Verification items for the finished model (mm, model axes). A direction names the side the tool comes from. Give positions to 0.01 mm unless a question says otherwise; leave off trailing zeros. Loops run counter-clockwise (first coordinate to the right, second up) from the corner with the lowest first, then second, coordinate; pieces in that order, holes last. Notation, with made-up numbers: (-19, 79) - (-4, 79) arc R5 cw to (-4, 86) - close; hole circle Ø1 at (21.5, 74.25). An arc over 180 degrees is marked (long way). Use one line per item in the form item = value.
```python
from build123d import *

# Parameters (mm, degrees)
HOLE_WIZARD_M6_1_D     = 5
HOLE_WIZARD_M6_1_DEPTH = 15
HOLE_WIZARD_M6_1_TIP   = 1.502151548
CHAMFER_1_SIZE         = 0.2


with BuildPart() as part:
    # 草图1 → 旋转1 (revolve)
    with BuildSketch(Plane.XY):
        Polygon((0, 0), (7.5, 0), (7.5, 70.5), (4.5, 70.5), (4.5, 72.5), (5, 72.5), (5, 76.267949192), (4, 80), (0, 80), align=None)
    revolve(axis=Axis((0, -1000, 0), (0, 1, 0)))

    # M6 螺纹孔1
    with Locations(Plane(origin=(0, 0, 0), x_dir=(-1, 0, 0), z_dir=(0, -1, 0))):
        with Locations((0, 0)):
            Hole(HOLE_WIZARD_M6_1_D / 2, depth=HOLE_WIZARD_M6_1_DEPTH)
            with Locations((0, 0, -(HOLE_WIZARD_M6_1_DEPTH + HOLE_WIZARD_M6_1_TIP / 2))):  # 118° drill point
                Cone(0, HOLE_WIZARD_M6_1_D / 2, HOLE_WIZARD_M6_1_TIP, mode=Mode.SUBTRACT)

    # 倒角1
    chamfer_1_edges = [part.edges().sort_by_distance(p)[0] for p in [
        (-7.5, 0, 0),
    ]]
    chamfer(chamfer_1_edges, length=CHAMFER_1_SIZE)


solid = part.part
```
1. Scan lines: probe 1 along Z at (x, y) = (0, 9.5); probe 2 along Y at (x, z) = (-5, -3.5); probe 3 along Z at (x, y) = (0, 75.5). Record each from-to range of solid material in increasing order.
Result set:
probe_1 = -7.5 to -2.5, 2.5 to 7.5
probe_2 = 0 to 70.5
probe_3 = -5 to 5
2. Draft check along Y on faces 1 (the flat face through (0, 0, 3)), 2 (the conical face through (3.97, 79.4, -1.25)), 3 (the cylindrical face through (-0.59, 71.51, -4.46)), 4 (the cylindrical face through (-0.54, 7.6, 2.44)). Enter one of: released by +Y, released by -Y, zero draft, split by the parting line, or undercut.
Result set:
face_1 = released by -Y
face_2 = released by +Y
face_3 = undercut
face_4 = zero draft
3. Tool access check on faces 5 (the flat face through (0, 70.5, 5)), 6 (the cylindrical face through (-1.08, 74.41, 4.88)), 7 (the cylindrical face through (-7.493, 35.842, -0.33)). Record the directions out of +Z, -Z, +X, -X, +Y, -Y that give a thin tool (end or side, any length) a straight path to the whole face; none if there is none.
Result set:
face_5 = none
face_6 = +Y
face_7 = +Y, -Y
4. Section check A-A, the plane y = 8.5. Record the cut outline in (x, z).
Result set:
outline = circle Ø15 at (0, 0); hole circle Ø5 at (0, 0)
5. Section check B-B, the plane y = 46.5. Record the cut outline in (x, z), then the cut area to 3 significant figures.
Result set:
outline = circle Ø15 at (0, 0)
area = 177 mm²
6. Depth check by flat-ended pin: pin 1 Ø1 at (x, y) = (4, 56.5) entering from +Z; pin 2 Ø2 at (x, z) = (-5.5, -5) entering from +Y; pin 3 Ø8 at (y, z) = (64, -3) entering from -X; pin 4 Ø6 at (x, y) = (5, 46.5) entering from +Z. Enter the tip coordinate at first touch or a pass-through.
Result set:
pin_1 = 6.63
pin_2 = 70.5
pin_3 = -7.5
pin_4 = 7.23
